Input: part model. Units: mm. Frame: model coordinates. A direction names the side the tool comes from. Give positions to 0.01 mm unless a question says otherwise; leave off trailing zeros. Loops run counter-clockwise (first coordinate to the right, second up) from the corner with the lowest first, then second, coordinate; pieces in that order, holes last. Notation, with made-up numbers: (-21, -8) -> (38, -8) arc R30 ccw to (38, 20) -> close; hole circle Ø8 at (26.5, 69). An arc over 180 degrees is marked (long way). Answer as a JSON object with one key per item and string values.
```python
from build123d import *

# Parameters (mm, degrees)
SKETCH1_W = 6
SKETCH1_H = 2


with BuildPart() as part:
    # Sketch1 → Revolve1 (revolve)
    with BuildSketch(Plane.XY, mode=Mode.PRIVATE) as revolve1_sk:
        Polygon((-12.5, 2), (-12.5, 0), (14.5, 0), (14.5, 3.125), (-12.5, 3.125), align=None)
        with Locations((-15.5, 1)):
            Rectangle(SKETCH1_W, SKETCH1_H)
        Polygon((14.5, 3.125), (14.5, 0), (18.5, 0), (18.5, 5), (14.5, 5), align=None)
    revolve(revolve1_sk.sketch.rotate(Axis((-18.5, 0, 0), (1, 0, 0)), 180), axis=Axis((-18.5, 0, 0), (1, 0, 0)))


solid = part.part
```
Q1. Access query for faces 1 (the cylindrical face through (-15, 0, 2)), 2 (the cylindrical face through (16, 5, 0)). Directions: +Z, -Z, +X, -X, +Y, -Y. A direction counts if a zero-diameter tool reaches every point of the face in a straight line with its end or side. Return the directions, or none.
Evaluation:
{"face 1": "-X", "face 2": "+X, -X"}
Q2. Section A-A, the plane y = 0. Return the cut outline in (x, z) (3 decimals), then the cut area to 3 significant figures.
Evaluation:
{"outline": "(-18.5, -2) -> (-12.5, -2) -> (-12.5, -3.125) -> (14.5, -3.125) -> (14.5, -5) -> (18.5, -5) -> (18.5, 5) -> (14.5, 5) -> (14.5, 3.125) -> (-12.5, 3.125) -> (-12.5, 2) -> (-18.5, 2) -> close", "area": "233 mm2"}
Q3. Pin query (flat end, axial travel): pin 1 (1 mm diameter, centred on y = 1.5, z = 3, fed in from -X); pin 2 (5 mm diameter, centred on x = 8, z = -1.5, fed in from -Y) (3 decimals); pin 3 (6 mm diameter, centred on x = 1, z = 0.5, fed in from +Y) (3 decimals). Return the tip coordinate at first contact, or that it passes through.
Evaluation:
{"pin 1": "stops at x = -12.5", "pin 2": "stops at y = -3.125", "pin 3": "stops at y = 3.125"}
Q4. Section C-C, the plane x = 16.5. Return the cut outline in (y, z).
Evaluation:
{"outline": "circle Ø10 at (0, 0)"}
Q5. Section D-D, the plane z = -2.5. Return the cut outline in (x, y) (3 decimals).
Evaluation:
{"outline": "(-12.5, -1.875) -> (14.5, -1.875) -> (14.5, -4.33) -> (18.5, -4.33) -> (18.5, 4.33) -> (14.5, 4.33) -> (14.5, 1.875) -> (-12.5, 1.875) -> close"}
Q6. Ray query, line 1 along X through (y, z) = (0.5, -3.5); line 2 along X through (y, z) = (2.5, -1.75); line 3 along Y through (x, z) = (-3.5, 1.25). Return the intervals inside material, ascending.
Evaluation:
{"line 1": "x = 14.5 to 18.5", "line 2": "x = -12.5 to 18.5", "line 3": "y = -2.86 to 2.86"}
